Can you work these out from the model? Positions are in its coordinate system, mm. Coordinates: 2 decimals unless noted, no trailing zeros. Answer as a JSON object with one key per item and string values.
Autodesk Inventor part; units mm, degrees
ref_plane "YZ Plane" through (0, 0, 0) normal (1, 0, 0) x (0, 1, 0)
ref_plane "XZ Plane" through (0, 0, 0) normal (0, 1, 0) x (-1, 0, 0)
ref_plane "XY Plane" through (0, 0, 0) normal (0, 0, 1) x (1, 0, 0)
sketch "スケッチ1" plane through (0, 0, 0) normal (0, 1, 0) x (-1, 0, 0)
  line L0 (0, 0) -> (-220, 0)
  line L1 (-220, 0) -> (-220, -35)
  line L2 (-220, -35) -> (0, -35)
  line L3 (0, -35) -> (0, 0)
  arc A0 (0, -35) -> (0, 0) centre (0, -17.5) ccw
  dimension "d0" = 220
  dimension "d1" = 35
  dimension "d2" = 17.5
extrude "押し出し1" add sketch "スケッチ1" along normal blind 3
sketch "スケッチ2" plane through (0, 3, 0) normal (0, 1, 0) x (1, 0, 0)
  line L0 (0, 17.5) -> (238.6526, 17.5)
  line L1 (0, 0) -> (220, 0)
  arc A0 (0, 35) -> (0, 0) centre (0, 17.5) ccw
  point P0 (30, 17.5)
  point P1 (40, 17.5)
  point P2 (50, 17.5)
  point P3 (60, 17.5)
  point P4 (70, 17.5)
  point P5 (80, 17.5)
  point P6 (90, 17.5)
  point P7 (100, 17.5)
  point P8 (110, 17.5)
  point P9 (120, 17.5)
  point P10 (130, 17.5)
  point P11 (140, 17.5)
  point P12 (150, 17.5)
  point P13 (160, 17.5)
  point P14 (170, 17.5)
  point P15 (180, 17.5)
  point P16 (190, 17.5)
  point P17 (200, 17.5)
  point P18 (210, 17.5)
  point P19 (-17.5, 17.5)
  dimension "d5" = 17.5
  dimension "d7" = 10
  dimension "d8" = 10
  dimension "d9" = 10
  dimension "d10" = 10
  dimension "d11" = 10
  dimension "d12" = 10
  dimension "d13" = 10
  dimension "d14" = 10
  dimension "d15" = 10
  dimension "d16" = 10
  dimension "d17" = 10
  dimension "d18" = 10
  dimension "d19" = 10
  dimension "d20" = 10
  dimension "d21" = 10
  dimension "d22" = 10
  dimension "d23" = 10
  dimension "d24" = 10
  dimension "d35" = 17.5
hole "穴1" at (30, 3, -17.5) at (40, 3, -17.5) at (50, 3, -17.5) at (60, 3, -17.5) at (70, 3, -17.5) at (80, 3, -17.5) at (90, 3, -17.5) at (100, 3, -17.5) at (110, 3, -17.5) at (120, 3, -17.5) at (130, 3, -17.5) at (140, 3, -17.5) at (150, 3, -17.5) at (160, 3, -17.5) at (170, 3, -17.5) at (180, 3, -17.5) at (190, 3, -17.5) at (200, 3, -17.5) at (210, 3, -17.5) direction (0, -1, 0) diameter 3.2 end through all
sketch "スケッチ3" plane through (0, 3, 0) normal (0, 1, 0) x (1, 0, 0)
  line L0 (220, 35) -> (0, 35)
  point P0 (0, 0)
  point P1 (0, 17.5)
  dimension "d36" = 17.5
hole "穴2" at (0, 3, -17.5) direction (0, -1, 0) diameter 8.5 end through all
sketch "スケッチ4" plane through (0, 3, 0) normal (0, 1, 0) x (1, 0, 0)
  circle A0 centre (0, 17.5) radius 12.5
  circle A1 centre (0, 17.5) radius 4.25
  line L0 (-6.6439, 17.5) -> (-13.0454, 17.5)
  line L1 (-13.0454, 17.5) -> (1.0104, 17.5)
  point P0 (0, 0)
  point P1 (0, 5)
  point P2 (12.5, 17.5)
  point P3 (0, 30)
  point P4 (-12.5, 17.5)
  dimension "d44" = 25
  dimension "d45" = 0
hole "穴3" at (0, 3, -5) at (12.5, 3, -17.5) at (0, 3, -30) at (-12.5, 3, -17.5) direction (0, -1, 0) diameter 2.459 end through all
properties part number "arm_plate1" material "アルミニウム 5052"
Item 1: Please list where these lines run through material, in increasing order: line 1 (Z direction, x = 0, y = 1.45); line 2 (Z direction, x = 30, y = 1.4); line 3 (Z direction, x = 12.5, y = 1.5).
Answers follow:
{"line 1": "z = -35 to -31.23, -28.77 to -21.75, -13.25 to -6.23, -3.77 to 0", "line 2": "z = -35 to -19.1, -15.9 to 0", "line 3": "z = -35 to -18.73, -16.27 to 0"}
Item 2: If we mould it in two halves opening along X, with no side actions, what happens to faces 1 (the flat face through (103, 0, -17)), 2 (the cylindrical face through (-17.496, 1.479, -17.115)), 3 (the cylindrical face through (-2.872, 1.479, -20.632))? For each: pulls with the +X half, pulls with the -X half, needs draft (parallel to the pull), parting line crosses it, or undercut.
Answers follow:
{"face 1": "needs draft", "face 2": "pulls with the -X half", "face 3": "undercut"}
Item 3: I'm going to push a flat-ended pin straight in: pin 1 (3 mm diameter, centred on x = 80, z = -17.5, fed in from -Y). Where does the tip first touch, or does it pass through?
Answers follow:
{"pin 1": "passes through"}
Item 4: I want a section at A-A, the plane y = 0.8. Give the number of separate pieces and of enclosed holes in the cut face, plus the area to 3 significant figures.
Answers follow:
{"separate pieces": "1", "enclosed holes": "24", "area": "7,950 mm^2"}
